The listing builds one solid part. Answer for the finished solid, in the listing's coordinates (mm). A direction names the side the tool comes from. Coordinates: 2 decimals unless noted, no trailing zeros. Order: outer loops, then holes, each group sorted by start corner. A loop starts at its lowest first (then second) coordinate and runs counter-clockwise, first axis right, second up. Notation, with made-up numbers: (4.25, 15.25) - (13.25, 15.25) arc R20 cw to (13.25, 34.25) - close; hole circle Ø10 at (-32, 51). An arc over 180 degrees is marked (long way). Use a Markdown table: item, result. Add a question column.
Item 1: Find the intervals of material crossed by line 1 along Y through (x, z) = (-0.5, 2.5); line 2 along Z through (x, y) = (2.25, -1.25) (3 decimals); line 3 along X through (y, z) = (-9.5, 1.8), in increasing order.
Item 2: For faces 5 (the flat face through (0, -7.938, 2)), 6 (the cylindrical face through (-0.033, -14.754, 1.415)), 7 (the flat face through (3.969, -4, 2)), 8 (the cylindrical face through (-0.516, -6.293, 3.958)), 9 (the flat face through (0, -3, 0)), determine the directions among +Z, -Z, +X, -X, +Y, -Y from which every point of the face is accessible in a straight line to the end or side of a thin tool.
Item 3: The part is cut by section B-B, the plane y = -8.5. Give the vertices of the cut face in (x, z) (3 decimals).
Item 4: The mould has two halves that part along Y. Classify faces 1 (the flat face through (-3.969, -4, 2)), 2 (the flat face through (0, 0, 3.175)), 3 (the flat face through (0, 7.938, 2)), 4 (the cylindrical face through (-0.31, 6.33, 3.96)): released by +Y, released by -Y, zero draft, split by the parting line, or undercut.
Item 5: The part is cut by section C-C, the plane z = 2.7. Give the vertices of the cut face in (x, y).
Item 6: Flat-ended cylindrical pins translate along their axes: P1, Ø1.6, axis at x = 0, z = 2, coming from the -Y side; P2, Ø1.5, axis at x = -1.5, y = -12.5, coming from the -Z side. Find the tip coordinate at first contact, or state that the pin passes through.
Item 7: The part is cut by section D-D, the plane z = 3.65. Give the vertices of the cut face in (x, y).
from build123d import *

# Parameters (mm, degrees)
F0_W     = 7.9375
F0_H     = 15.875
F0_R     = 2.38125
F1_DEPTH = 3.175
F2_DEPTH = 4.7625
F4_DEPTH = 1.5875
F6_R     = 1.5875
F7_DEPTH = 4.7625


with BuildPart() as f1:
    # F0 (on Top) → F1 (new body)
    with BuildSketch(Plane.XY):
        Rectangle(F0_W, F0_H)
        with Locations((0, -3.96875)):
            Circle(F0_R, mode=Mode.SUBTRACT)
        with Locations((0, 3.96875)):
            Circle(F0_R, mode=Mode.SUBTRACT)
    extrude(amount=F1_DEPTH)

    # F0 (on Top) → F2 (join)
    with BuildSketch(Plane.XY):
        with Locations((0, 3.96875)):
            Circle(F0_R)
        with Locations((0, -3.96875)):
            Circle(F0_R)
    extrude(amount=F2_DEPTH)

    # F3 (on face) → F4 (join)
    with BuildSketch(Plane(origin=(-3.96875, 0, 0), x_dir=(0, -1, 0), z_dir=(-1, 0, 0))):
        Polygon((7.9375, 3.175), (7.9375, 0), (11.1125, 0), (11.1125, 2.38125), (11.1125, 3.175), align=None)
        with BuildLine():
            Line((11.1125, 2.38125), (11.1125, 0))
            Line((11.1125, 0), (13.49375, 0))
            ThreePointArc((13.49375, 0), (11.809952, 0.697452), (11.1125, 2.38125))
        make_face()
        with BuildLine():
            Line((11.1125, 3.175), (11.1125, 2.38125))
            ThreePointArc((11.1125, 2.38125), (11.146793, 2.783924), (11.248686, 3.175))
            Line((11.248686, 3.175), (11.1125, 3.175))
        make_face()
        with BuildLine():
            ThreePointArc((11.248686, 3.175), (11.146793, 2.783924), (11.1125, 2.38125))
            ThreePointArc((11.1125, 2.38125), (11.809952, 0.697452), (13.49375, 0))
            ThreePointArc((13.49375, 0), (15.177548, 0.697452), (15.875, 2.38125))
            ThreePointArc((15.875, 2.38125), (13.896424, 4.728207), (11.248686, 3.175))
        make_face()
    extrude(amount=-F4_DEPTH)

    # F5: F1 across plane


with BuildPart() as f1_1:
    add(f1.part)
    add(f1.part.mirror(Plane.YZ))

    # F6 (on face) → F7 (join)
    with BuildSketch(Plane.YZ.offset(-2.38125)):
        with Locations((-13.49375, 2.38125)):
            Circle(F6_R)
    extrude(amount=F7_DEPTH)


solid = f1_1.part
Solution:
| question | item | result |
|---|---|---|
| 1 | line 1 | y = -15.08 to -11.91, -7.94 to 7.94 |
| 1 | line 2 | z = 0 to 3.175 |
| 1 | line 3 | x = -3.97 to -2.38, 2.38 to 3.97 |
| 2 | face 5 | +Z, -Z |
| 2 | face 6 | none |
| 2 | face 7 | +Z, -Z, +X, +Y, -Y |
| 2 | face 8 | +Z |
| 2 | face 9 | -Z, +X, -X, +Y, -Y |
| 3 | outline | (-3.969, 0) - (-2.381, 0) - (-2.381, 3.175) - (-3.969, 3.175) - close; (2.381, 0) - (3.969, 0) - (3.969, 3.175) - (2.381, 3.175) - close |
| 4 | face 1 | zero draft |
| 4 | face 2 | undercut |
| 4 | face 3 | released by +Y |
| 4 | face 4 | undercut |
| 5 | outline | (-3.97, -15.85) - (-2.38, -15.85) - (-2.38, -15.05) - (2.38, -15.05) - (2.38, -15.85) - (3.97, -15.85) - (3.97, 7.94) - (-3.97, 7.94) - close; hole (-2.38, -11.94) - (2.38, -11.94) - (2.38, -7.94) - (-2.38, -7.94) - close |
| 6 | P1 | stops at y = -15.08 |
| 6 | P2 | stops at z = 0.81 |
| 7 | outline | (-3.97, -15.51) - (-2.38, -15.51) - (-2.38, -14.45) - (2.38, -14.45) - (2.38, -15.51) - (3.97, -15.51) - (3.97, -11.48) - (2.38, -11.48) - (2.38, -12.54) - (-2.38, -12.54) - (-2.38, -11.48) - (-3.97, -11.48) - close; circle Ø4.76 at (0, -3.97); circle Ø4.76 at (0, 3.97) |
